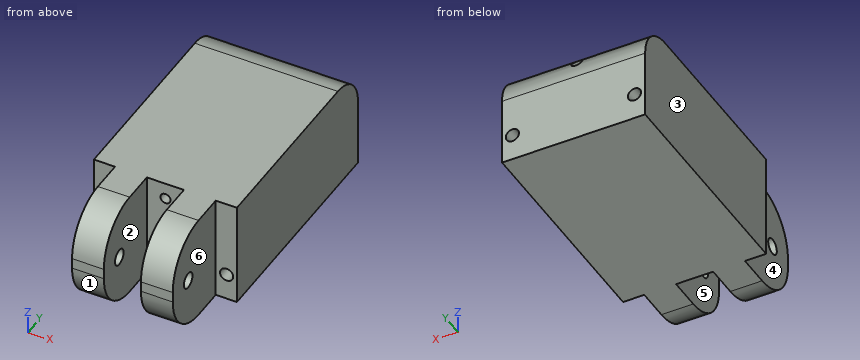
from build123d import *

# Parameters (mm, degrees)
PAD_DEPTH       = 20
FILLET_R        = 7
SKETCH001_R     = 1.5
POCKET_DEPTH    = 23.001
SKETCH002_R     = 1.25
SKETCH002_R_2   = 0.961399
POCKET001_DEPTH = 42.236626
FILLET001_R     = 9
FILLET002_R     = 9
FILLET003_R     = 9
FILLET004_R     = 9


with BuildPart() as part:
    # Sketch → Pad (new body)
    with BuildSketch(Plane.XY):
        Polygon((-31.448001, 43.877556), (-31.448001, 36.642305), (-31.448001, 1.642305), (-27.448001, 1.642283), (-27.448001, -13.357717), (-21.448001, -13.357717), (-21.448001, 1.642283), (-14.448001, 1.642283), (-14.448001, -13.357717), (-8.448001, -13.357717), (-8.448001, 1.64193), (-4.448001, 1.64193), (-4.448001, 36.64193), (-4.448001, 43.877556), align=None)
    extrude(amount=PAD_DEPTH)

    # Fillet
    fillet_edges = [part.edges().sort_by_distance(p)[0] for p in [
        (-17.948001, 43.877556, 20),
    ]]
    fillet(fillet_edges, radius=FILLET_R)

    # Sketch001 (on Face15 of Fillet) → Pocket (cut, through all)
    with BuildSketch(Plane.YZ.offset(-8.448001)):
        with Locations((-7.970362, 9.805142)):
            Circle(SKETCH001_R)
    extrude(amount=-POCKET_DEPTH, mode=Mode.SUBTRACT)

    # Sketch002 (on Face16 of Pocket) → Pocket001 (cut, through all)
    with BuildSketch(Plane.XZ.offset(-1.64193)):
        with Locations((-6.398813, 5.068225)):
            Circle(SKETCH002_R)
        with Locations((-29.421452, 5)):
            Circle(SKETCH002_R)
        with Locations((-17.935286, 16.84268)):
            Circle(SKETCH002_R_2)
    extrude(amount=-POCKET001_DEPTH, mode=Mode.SUBTRACT)

    # Fillet001
    fillet001_edges = [part.edges().sort_by_distance(p)[0] for p in [
        (-11.448001, -13.357717, 20),
    ]]
    fillet(fillet001_edges, radius=FILLET001_R)

    # Fillet002
    fillet002_edges = [part.edges().sort_by_distance(p)[0] for p in [
        (-24.448001, -13.357717, 20),
    ]]
    fillet(fillet002_edges, radius=FILLET002_R)

    # Fillet003
    fillet003_edges = [part.edges().sort_by_distance(p)[0] for p in [
        (-11.448001, -13.357717, 0),
    ]]
    fillet(fillet003_edges, radius=FILLET003_R)

    # Fillet004
    fillet004_edges = [part.edges().sort_by_distance(p)[0] for p in [
        (-24.448001, -13.357717, 0),
    ]]
    fillet(fillet004_edges, radius=FILLET004_R)


solid = part.part
Geometry check sheet. Reference: the model listing, model coordinates, mm. Face numbers are marked on the shaded views. A direction names the side the tool comes from. Round coordinates to 2 decimals unless told otherwise and drop trailing zeros. Loops run counter-clockwise (first coordinate to the right, second up) from the corner with the lowest first, then second, coordinate; pieces in that order, holes last. Notation, with made-up numbers: (49.25, -15.5) -> (57.25, -15.5) arc R28 cw to (57.25, 22.5) -> close; hole circle Ø2 at (-32, -23.5). An arc over 180 degrees is marked (long way). Answer as a JSON object with one key per item and string values. Group by question number.
Item 1: Cross-section at C-C, the plane x = -20. Record the cut outline in (y, z), plus the area to 3 significant figures.
Item 2: Cross-section at B-B, the plane x = -26.25. Record the cut outline in (y, z), plus the area to 3 significant figures.
Item 3: Cross-section at A-A, the plane y = -3. Record the cut outline in (x, z).
Item 4: Depth check by flat-ended pin: pin 1 Ø7.5 at (y, z) = (-6, 9.5) entering from -X; pin 2 Ø3 at (x, z) = (-29, 11.5) entering from -Y; pin 3 Ø4.5 at (y, z) = (-8.5, 10) entering from +X. Enter the tip coordinate at first touch or a pass-through.
Item 5: Thickness scan on line 1 along X through (y, z) = (14, 5); line 2 along X through (y, z) = (1.5, 3); line 3 along Z through (x, y) = (-18.25, 34). Record the ranges inside material, lowest first.
Item 6: Cross-section at D-D, the plane y = 35. Record the cut outline in (x, z).
Item 7: Set-up check for the marked faces 4, 5 and 6: record each of +Z, -Z, +X, -X, +Y, -Y from which the full face is reachable in a straight line by a thin tool's end or side.
Item 8: Release check for a two-part mould opening along X. For the marked faces 1, 2 and 3 record: pulls with the +X half, pulls with the -X half, needs draft (parallel to the pull), parting line crosses it, or undercut.
Determined:
{
 "1": {"outline": "(1.64, 0) -> (43.88, 0) -> (43.88, 13) arc R7 ccw to (36.88, 20) -> (1.64, 20) -> close", "area": "834 mm²"},
 "2": {"outline": "(-13.36, 9) arc R9 ccw to (-4.36, 0) -> (43.88, 0) -> (43.88, 13) arc R7 ccw to (36.88, 20) -> (-4.36, 20) arc R9 ccw to (-13.36, 11) -> close; hole circle Ø3 at (-7.97, 9.81)", "area": "1,090 mm²"},
 "3": {"outline": "(-27.45, 0) -> (-21.45, 0) -> (-21.45, 20) -> (-27.45, 20) -> close; (-14.45, 0) -> (-8.45, 0) -> (-8.45, 20) -> (-14.45, 20) -> close"},
 "4": {"pin 1": "stops at x = -27.45", "pin 2": "stops at y = 1.64", "pin 3": "stops at x = -8.45"},
 "5": {"line 1": "x = -31.45 to -30.67, -28.17 to -7.65, -5.15 to -4.45", "line 2": "x = -27.45 to -21.45, -14.45 to -8.45", "line 3": "z = 0 to 15.93, 17.75 to 20"},
 "6": {"outline": "(-31.45, 0) -> (-4.45, 0) -> (-4.45, 20) -> (-31.45, 20) -> close; hole circle Ø2.5 at (-29.42, 5); hole circle Ø1.92 at (-17.94, 16.84); hole circle Ø2.5 at (-6.4, 5.07)"},
 "7": {"face 4": "+Z, -Z, -X, -Y", "face 5": "+Z, -Z, -Y", "face 6": "+Z, -Z, +X, -Y"},
 "8": {"face 1": "needs draft", "face 2": "undercut", "face 3": "pulls with the -X half"}
}
